from build123d import *

# Parameters (mm, degrees)
SKETCH3_W           = 228
SKETCH3_H           = 914
BOSS_EXTRUDE2_DEPTH = 127
SKETCH4_W           = 63
SKETCH4_H           = 152
CUT_EXTRUDE1_DEPTH  = 127
SKETCH6_R           = 26
CUT_EXTRUDE2_DEPTH  = 127


with BuildPart() as part:
    # Sketch3 → Boss-Extrude2 (new body)
    with BuildSketch(Plane.XY):
        Rectangle(SKETCH3_W, SKETCH3_H)
    extrude(amount=BOSS_EXTRUDE2_DEPTH)

    # Sketch4 → Cut-Extrude1 (cut)
    with BuildSketch(Plane(origin=(114, 0, 0), x_dir=(0, 0, -1), z_dir=(1, 0, 0))):
        with Locations((-63.5, 305)):
            Rectangle(SKETCH4_W, SKETCH4_H)
    extrude(amount=-CUT_EXTRUDE1_DEPTH, mode=Mode.SUBTRACT)

    # Sketch6 → Cut-Extrude2 (cut)
    with BuildSketch(Plane.XY):
        with Locations((50.5, 305)):
            Circle(SKETCH6_R)
    extrude(amount=CUT_EXTRUDE2_DEPTH, mode=Mode.SUBTRACT)


solid = part.part
Here's how the part is built. I have some questions about the finished solid (model axes, mm). A direction names the side the tool comes from. Coordinates: 2 decimals unless noted, no trailing zeros. Write each loop counter-clockwise with the first axis right and the second up, starting at its lowest first coordinate (ties: lowest second). Pieces come first, ordered by that corner, then holes.
1) If we section it at C-C (z = 56): List the corners of the cut face in (x, y) for me, plus the area to 3 significant figures.
Filled in:
outline: (-114, -457) - (114, -457) - (114, 229) - (-13, 229) - (-13, 381) - (114, 381) - (114, 457) - (-114, 457) - close
area: 189,000 mm2
2) If we section it at B-B (x = 50.5): List the corners of the cut face in (y, z) for me.
Filled in:
outline: (-457, 0) - (279, 0) - (279, 32) - (229, 32) - (229, 95) - (279, 95) - (279, 127) - (-457, 127) - close; (331, 0) - (457, 0) - (457, 127) - (331, 127) - (331, 95) - (381, 95) - (381, 32) - (331, 32) - close
3) If we section it at A-A (y = 305): List the corners of the cut face in (x, z) for me, plus the area to 3 significant figures.
Filled in:
outline: (-114, 0) - (24.5, 0) - (24.5, 32) - (-13, 32) - (-13, 95) - (24.5, 95) - (24.5, 127) - (-114, 127) - close; (76.5, 0) - (114, 0) - (114, 32) - (76.5, 32) - close; (76.5, 95) - (114, 95) - (114, 127) - (76.5, 127) - close
area: 17,600 mm2
4) If I drill on line 1 (Y direction, x = 50, z = 14); line 2 (X direction, y = 305, z = 24.5); line 3 (X direction, y = 302, z = 29.5), over which ranges is the centre line in solid material (lowest first)?
Filled in:
line 1: y = -457 to 279, 331 to 457
line 2: x = -114 to 24.5, 76.5 to 114
line 3: x = -114 to 24.67, 76.33 to 114
5) Which directions (+Z, -Z, +X, -X, +Y, -Y) give clear straight access to the entire face, cutting with the end or side of a thin tool? Please do faces 1 (the face through (44.86, 279.62, 110.78)), 2 (the face through (80, 304, 95)).
Filled in:
face 1: +Z, -Z
face 2: +X
6) Thinking about a two-plate mould opening in Y: for faces 3 (the face through (-13, 306, 64)), 4 (the face through (-2, -457, 63)), 5 (the face through (114, -6, 63)), which applies, +Y half, -Y half, draft (parallel to the pull), parting line (faces both ways), or undercut?
Filled in:
face 3: undercut
face 4: -Y half
face 5: draft
